Geometry check sheet. Reference: the model listing, model coordinates, mm. Face numbers are marked on the shaded views. Round coordinates to 2 decimals unless told otherwise and drop trailing zeros. Loops run counter-clockwise (first coordinate to the right, second up) from the corner with the lowest first, then second, coordinate; pieces in that order, holes last. Notation, with made-up numbers: M 66,20.25 L 71,20.25 A13 ccw 71,24.25 Z; hole C 30,3 d6. An arc over 180 degrees is marked long. Use one line per item in the form item = value. Start each with the question number.
1. Cross-section at D-D (x = 18). Record the boundary of the cut face in (y, z).
2. Cross-section at C-C (z = 5.5). Record the boundary of the cut face in (x, y).
3. Draft check along X on the marked faces 1, 2, 3 and 4. Enter one of: pulls with the +X half, pulls with the -X half, needs draft (parallel to the pull), parting line crosses it, or undercut.
4. Material ranges on line 1 (X direction, y = -26.5, z = 14.25); line 2 (Y direction, x = 10.5, z = 12.75); line 3 (X direction, y = -28.5, z = 4.5), recorded low to high.
5. Cross-section at B-B (y = -22). Record the boundary of the cut face in (x, z).
6. Go/stop test with flat-tipped pins: pin 1 (8 mm diameter, centred on x = 24, z = 8.5, fed in from +Y); pin 2 (6 mm diameter, centred on x = -7, z = 7.5, fed in from +Y); pin 3 (1 mm diameter, centred on y = -20.5, z = 9, fed in from +X). Record where each tip stops, or that it passes through.
7. Cross-section at A-A (x = 5.5). Record the boundary of the cut face in (y, z), then the cut area to 3 significant figures.
```python
from build123d import *

# Parameters (mm, degrees)
F0_W     = 50
F0_H     = 70
F1_DEPTH = 15
F2_R     = 6
F3_DEPTH = 25
F4_R     = 8
F5_DEPTH = 50.001
F6_R     = 3.5
F7_DEPTH = 15.001
F8_W     = 12
F8_H     = 25
F9_DEPTH = 15
F10_R    = 10


# Not quite as in the source:
# - a feature names something its author has since deleted; it is built from what else it names


with BuildPart() as f1:
    # F0 (on Top) → F1 (new body)
    with BuildSketch(Plane.XY):
        with Locations((6.2123397365, -48.3642113331)):
            Rectangle(F0_W, F0_H)
    extrude(amount=F1_DEPTH)

    # F2 (on face) → F3 (cut)
    with BuildSketch(Plane.XY.offset(15)):
        with Locations((6.2123397365, -25.3642113331)):
            Circle(F2_R)
    extrude(amount=-F3_DEPTH, mode=Mode.SUBTRACT)

    # F4 (on face) → F5 (cut, through all)
    with BuildSketch(Plane.YZ.offset(31.2123397365)):
        with Locations((-58.3642113331, 15)):
            Circle(F4_R)
    extrude(amount=-F5_DEPTH, mode=Mode.SUBTRACT)

    # F6 (on face) → F7 (cut, through all)
    with BuildSketch(Plane(origin=(0, 0, 0), x_dir=(1, 0, 0), z_dir=(0, 0, -1))):
        with Locations((6.2123397365, 43.3642113331)):
            Circle(F6_R)
        with Locations((6.2123397365, 73.3642113331)):
            Circle(F6_R)
    extrude(amount=-F7_DEPTH, mode=Mode.SUBTRACT)

    # F8 (on face) → F9 (cut, through all)
    with BuildSketch(Plane.XY.offset(15)):
        with Locations((25.2123397365, -25.8642113331)):
            Rectangle(F8_W, F8_H)
        with Locations((-12.7876602635, -25.8642113331)):
            Rectangle(F8_W, F8_H)
    extrude(amount=-F9_DEPTH, mode=Mode.SUBTRACT)

    # F10
    f10_edges = [f1.edges().sort_by_distance(p)[0] for p in [
        (19.21234, -13.364211, 7.5),
        (-6.78766, -13.364211, 7.5),
        (-6.78766, -38.364211, 7.5),
        (19.21234, -38.364211, 7.5),
    ]]
    fillet(f10_edges, radius=F10_R)


solid = f1.part
```
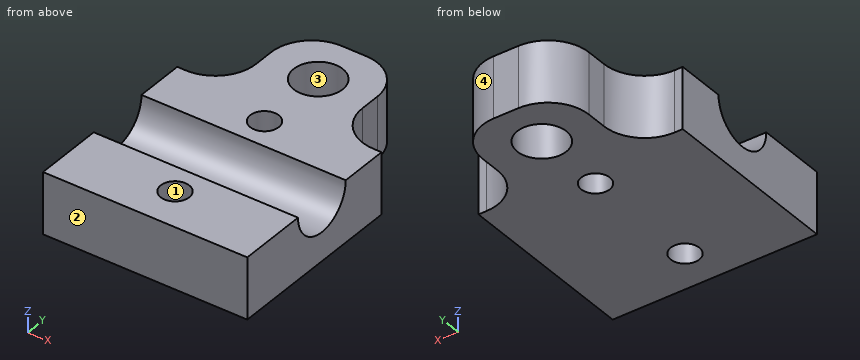
Reported:
q1.outline = M -83.36,0 L -18.59,0 L -18.59,15 L -50.36,15 A8 cw -66.36,15 L -83.36,15 Z
q2.outline = M -18.79,-83.36 L 31.21,-83.36 L 31.21,-38.36 L 29.21,-38.36 A10 cw 19.21,-28.36 L 19.21,-23.36 A10 ccw 9.21,-13.36 L 3.21,-13.36 A10 ccw -6.79,-23.36 L -6.79,-28.36 A10 cw -16.79,-38.36 L -18.79,-38.36 Z; hole C 6.21,-25.36 d12; hole C 6.21,-73.36 d7; hole C 6.21,-43.36 d7
q3.face_1 = undercut
q3.face_2 = needs draft
q3.face_3 = undercut
q3.face_4 = pulls with the +X half
q4.line_1 = -6.79 to 0.32, 12.1 to 19.21
q4.line_2 = -83.36 to -66.04, -50.69 to -29.56, -21.17 to -13.45
q4.line_3 = -6.79 to 1.1, 11.33 to 19.21
q5.outline = M -6.69,0 L 1.24,0 L 1.24,15 L -6.69,15 Z; M 11.18,0 L 19.12,0 L 19.12,15 L 11.18,15 Z
q6.pin_1 = -32.25
q6.pin_2 = -16.44
q6.pin_3 = 18.93
q7.outline = M -83.36,0 L -76.79,0 L -76.79,15 L -83.36,15 Z; M -69.94,0 L -46.79,0 L -46.79,15 L -50.36,15 A8 cw -66.36,15 L -69.94,15 Z; M -39.94,0 L -31.32,0 L -31.32,15 L -39.94,15 Z; M -19.41,0 L -13.36,0 L -13.36,15 L -19.41,15 Z
q7.area = 565 mm²
